```python
from build123d import *

# Parameters (mm, degrees)
BOSS_EXTRUDE1_DEPTH = 41.4
FILLET1_R           = 10


with BuildPart() as part:
    # Sketch1 → Boss-Extrude1 (new body)
    with BuildSketch(Plane(origin=(0, 0, 0), x_dir=(0, 1, 0), z_dir=(0, 0, 1))):
        with BuildLine():
            ThreePointArc((0, 0), (49.49489115, 7.831876421), (98.9897823, 0))
            ThreePointArc((98.9897823, 0), (121.763014729, -44.663014729), (77.1, -67.436247159))
            ThreePointArc((77.1, -67.436247159), (49.49489115, -63.068123579), (21.8897823, -67.436247159))
            ThreePointArc((21.8897823, -67.436247159), (-22.773232429, -44.663014729), (0, 0))
        make_face()
    extrude(amount=BOSS_EXTRUDE1_DEPTH)

    # Fillet1
    fillet1_edges = [part.edges().sort_by_distance(p)[0] for p in [
        (44.663014729, 121.763014729, 41.4),
        (-7.831876421, 49.49489115, 41.4),
        (44.663014729, -22.773232429, 41.4),
        (-7.831876421, 49.49489115, 0),
        (44.663014729, 121.763014729, 0),
        (63.068123579, 49.49489115, 0),
        (44.663014729, -22.773232429, 0),
        (63.068123579, 49.49489115, 41.4),
    ]]
    fillet(fillet1_edges, radius=FILLET1_R)


solid = part.part
```
For this review, take the finished solid that the model builds, in its own axes (mm). Coordinates: 2 decimals unless noted, no trailing zeros. Loops run counter-clockwise (first coordinate to the right, second up) from the corner with the lowest first, then second, coordinate; pieces in that order, holes last.
1. For line 1 (Y direction, x = 52, z = 21.5); line 2 (Y direction, x = 17, z = 17.5); line 3 (X direction, y = 109.5, z = 15), list the stretches that pass through material, from the lowest coordinate up.
2. Add section A-A, the plane z = 22.5. Give the boundary of the cut face in (x, y), then the cut area to 3 significant figures.
3. Mouldability with a two-part tool opening along Y and no side actions: class faces 1 (the cylindrical face through (-7.83, 48.79, 20.55)), 2 (the flat face through (30, 50, 41.4)), 3 (the cylindrical face through (63.07, 49.89, 20.55)) as +Y half, -Y half, draft (parallel to the pull), parting line (faces both ways), or undercut.
4. Insertion check: P1, Ø6, axis at y = 32.5, z = 33, coming from the -X side; P2, Ø3, axis at y = 65.5, z = 35, coming from the -X side; P3, Ø10, axis at y = -3.5, z = 24, coming from the +X side; P4, Ø10, axis at x = 29, y = 4, coming from the -Z side. Each pin has a flat end and moves straight along its axis. Give the tip position at first contact, or say it passes through.
Result:
1. line 1: y = -19.43 to 118.42
1. line 2: y = -20.32 to 119.31
1. line 3: x = 5.5 to 61.94
2. outline: (0, 0) arc R35.45 ccw to (67.44, 21.89) arc R89.41 cw to (67.44, 77.1) arc R35.45 ccw to (0, 98.99) arc R160.31 ccw to start
2. area: 9,510 mm2
3. face 1: parting line
3. face 2: draft
3. face 3: undercut
4. P1: stops at x = -7.19
4. P2: stops at x = -6.84
4. P3: stops at x = 67.89
4. P4: stops at z = 0
